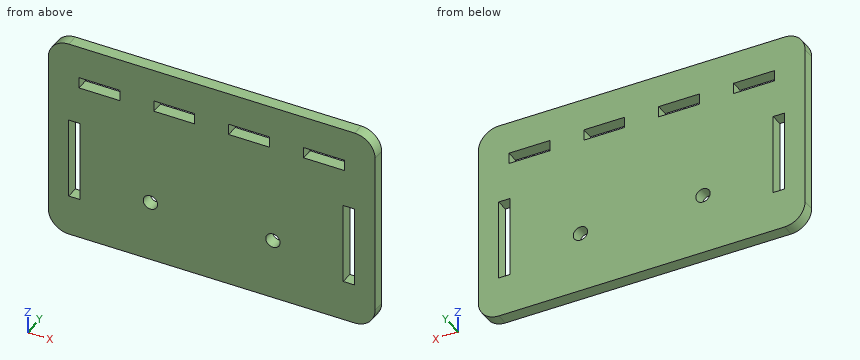
from build123d import *

# Parameters (mm, degrees)
SKETCH1_W           = 80
SKETCH1_H           = 50
SKETCH1_W_2         = 10
SKETCH1_H_2         = 2.7
SKETCH1_W_3         = 2.8
SKETCH1_H_3         = 20
BOSS_EXTRUDE1_DEPTH = 3
SKETCH2_R           = 1.75
CUT_EXTRUDE1_DEPTH  = 3
FILLET1_R           = 5


with BuildPart() as part:
    # Sketch1 → Boss-Extrude1 (new body)
    with BuildSketch(Plane(origin=(0, 0, 0), x_dir=(1, 0, 0), z_dir=(0, 1, 0))):
        Rectangle(SKETCH1_W, SKETCH1_H)
        with Locations((-9.17, -15.65)):
            Rectangle(SKETCH1_W_2, SKETCH1_H_2, mode=Mode.SUBTRACT)
        with Locations((-27.5, -15.65)):
            Rectangle(SKETCH1_W_2, SKETCH1_H_2, mode=Mode.SUBTRACT)
        with Locations((9.16, -15.65)):
            Rectangle(SKETCH1_W_2, SKETCH1_H_2, mode=Mode.SUBTRACT)
        with Locations((27.49, -15.65)):
            Rectangle(SKETCH1_W_2, SKETCH1_H_2, mode=Mode.SUBTRACT)
        with Locations((-33.6, 5)):
            Rectangle(SKETCH1_W_3, SKETCH1_H_3, mode=Mode.SUBTRACT)
        with Locations((33.6, 5)):
            Rectangle(SKETCH1_W_3, SKETCH1_H_3, mode=Mode.SUBTRACT)
    extrude(amount=BOSS_EXTRUDE1_DEPTH)

    # Sketch2 → Cut-Extrude1 (cut)
    with BuildSketch(Plane(origin=(0, 3, 0), x_dir=(1, 0, 0), z_dir=(0, 1, 0))):
        with Locations(Location((15, 10, 0), (0, 0, 270))):
            Circle(SKETCH2_R)
        with Locations(Location((-15, 10, 0), (0, 0, 270))):
            Circle(SKETCH2_R)
    extrude(amount=-CUT_EXTRUDE1_DEPTH, mode=Mode.SUBTRACT)

    # Fillet1
    fillet1_edges = [part.edges().sort_by_distance(p)[0] for p in [
        (-40, 1.5, -25),
        (40, 1.5, -25),
        (40, 1.5, 25),
        (-40, 1.5, 25),
    ]]
    fillet(fillet1_edges, radius=FILLET1_R)


solid = part.part
Read the model definition and answer for the solid it produces. Units are mm, in the model's axes. Give positions to 0.01 mm unless a question says otherwise; leave off trailing zeros. Write each loop counter-clockwise with the first axis right and the second up, starting at its lowest first coordinate (ties: lowest second). Pieces come first, ordered by that corner, then holes. Notation, with made-up numbers: (21, -39.5) -> (74, -39.5) arc R25 cw to (74, -3.5) -> close; hole circle Ø6 at (68, -29). An arc over 180 degrees is marked (long way). Answer as a JSON object with one key per item and string values. Group by question number.
1) Find section D-D (z = -2.5). Write down the section's boundary in (x, y), and give its area (3 significant figures).
2) Find section C-C (y = 1). Count the separate pieces of the cut face and the enclosed holes in it, and give its area (3 significant figures).
3) Find section A-A (x = -24). Write down the section's boundary in (y, z).
4) Find section B-B (z = -10). Write down the section's boundary in (x, y).
5) Consider L1, parallel to X at y = 1.5, z = -10; L2, parallel to X at y = 2.25, z = -7; L3, parallel to Z at x = -24, y = 2.3. Determine where each line is inside the solid, lowest interval first. Write a range as from..to.
Values follow:
{
 "1": {"outline": "(-40, 0) -> (-35, 0) -> (-35, 3) -> (-40, 3) -> close; (-32.2, 0) -> (32.2, 0) -> (32.2, 3) -> (-32.2, 3) -> close; (35, 0) -> (40, 0) -> (40, 3) -> (35, 3) -> close", "area": "223 mm2"},
 "2": {"separate pieces": "1", "enclosed holes": "8", "area": "3,740 mm2"},
 "3": {"outline": "(0, -25) -> (3, -25) -> (3, 14.3) -> (0, 14.3) -> close; (0, 17) -> (3, 17) -> (3, 25) -> (0, 25) -> close"},
 "4": {"outline": "(-40, 0) -> (-35, 0) -> (-35, 3) -> (-40, 3) -> close; (-32.2, 0) -> (-16.75, 0) -> (-16.75, 3) -> (-32.2, 3) -> close; (-13.25, 0) -> (13.25, 0) -> (13.25, 3) -> (-13.25, 3) -> close; (16.75, 0) -> (32.2, 0) -> (32.2, 3) -> (16.75, 3) -> close; (35, 0) -> (40, 0) -> (40, 3) -> (35, 3) -> close"},
 "5": {"L1": "x = -40..-35, -32.2..-16.75, -13.25..13.25, 16.75..32.2, 35..40", "L2": "x = -40..-35, -32.2..32.2, 35..40", "L3": "z = -25..14.3, 17..25"}
}
